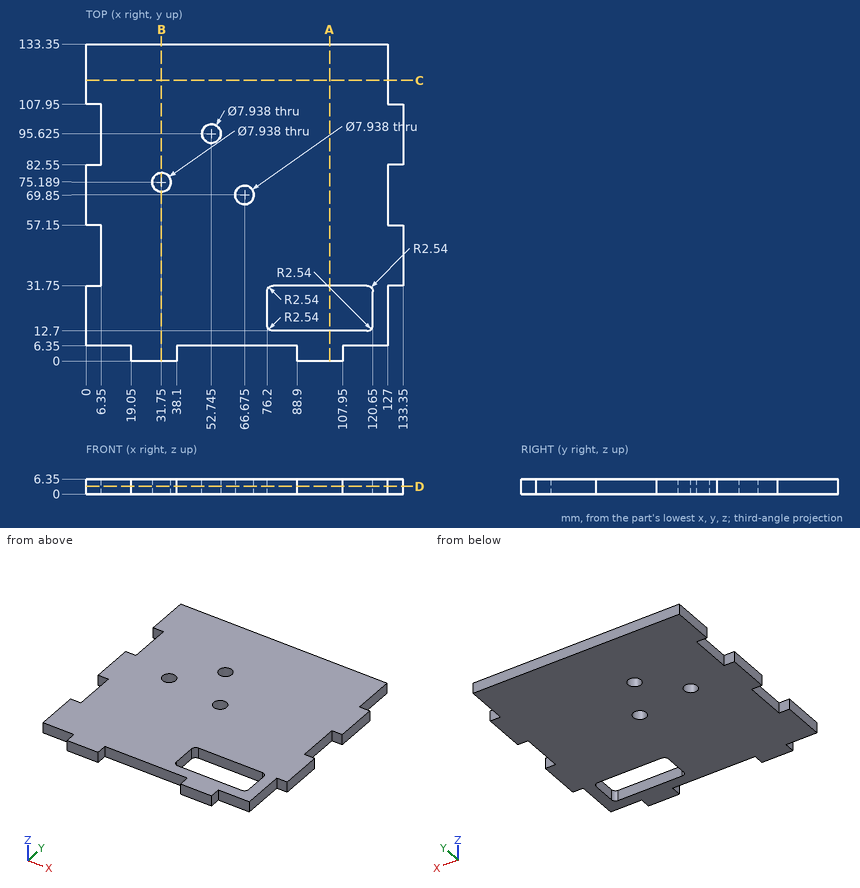
Input: dimensioned drawing with shaded views. Units: mm. Origin: part minimum x, y, z. Round coordinates to 2 decimals unless told otherwise and drop trailing zeros. Write each loop counter-clockwise with the first axis right and the second up, starting at its lowest first coordinate (ties: lowest second). Pieces come first, ordered by that corner, then holes. Notation, with made-up numbers: (-23.5, -3) -> (-12.5, -3) arc R21 cw to (-12.5, 24) -> close; hole circle Ø5 at (51, -23.75). An arc over 180 degrees is marked (long way). Use CSV: the item, a comma, the result in double quotes. Start each with the question number.
Q1. Line query: L1, parallel to X at y = 28, z = 1.5; L2, parallel to Y at x = 116, z = 2.5; L3, parallel to X at y = 70, z = 1.25. Output: solid intervals per line, ascending.
Q2. Section B-B (x = 31.75). Return loops of the section in (y, z).
Q3. Section C-C (y = 118). Return loops of the section in (x, z).
Q4. First-contact query: pin 1 Ø3 at (y, z) = (90, 4) entering from -X; pin 2 Ø7 at (x, y) = (66.675, 69.85) entering from -Z; pin 3 Ø3 at (x, z) = (130.5, 3) entering from +Y; pin 4 Ø1.5 at (y, z) = (66, 1) entering from +X. Flat tips, straight axial feed; report the tip coordinate or a pass-through.
Q5. Section D-D (z = 3.25). Give the number of separate pieces and of enclosed holes in the cut face, plus the area to 3 significant figures.
Q6. Section A-A (x = 102.5). Return loops of the section in (y, z).
Result sheet:
1,L1,"0 to 76.2, 120.65 to 127"
1,L2,"6.35 to 12.7, 31.75 to 133.35"
1,L3,"0 to 62.71, 70.64 to 127"
2,outline,"(0, 0) -> (71.22, 0) -> (71.22, 6.35) -> (0, 6.35) -> close; (79.16, 0) -> (133.35, 0) -> (133.35, 6.35) -> (79.16, 6.35) -> close"
3,outline,"(0, 0) -> (127, 0) -> (127, 6.35) -> (0, 6.35) -> close"
4,pin 1,"x = 6.35"
4,pin 2,"through"
4,pin 3,"y = 107.95"
4,pin 4,"x = 127"
5,separate pieces,"1"
5,enclosed holes,"4"
5,area,"15,400 mm²"
6,outline,"(0, 0) -> (12.7, 0) -> (12.7, 6.35) -> (0, 6.35) -> close; (31.75, 0) -> (133.35, 0) -> (133.35, 6.35) -> (31.75, 6.35) -> close"
